Print and shaded views of the part. All mm, measured from the part's lowest x, y and z. A direction names the side the tool comes from. Give positions to 0.01 mm unless a question says otherwise; leave off trailing zeros. Order: outer loops, then holes, each group sorted by start corner. A loop starts at its lowest first (then second) coordinate and runs counter-clockwise, first axis right, second up. Notation, with made-up numbers: (10.5, -3.5) - (46.5, -3.5) arc R21 ccw to (46.5, 25.5) - close; hole circle Ø7 at (16, -36). An arc over 180 degrees is marked (long way). Answer in a Markdown table with one row per item.
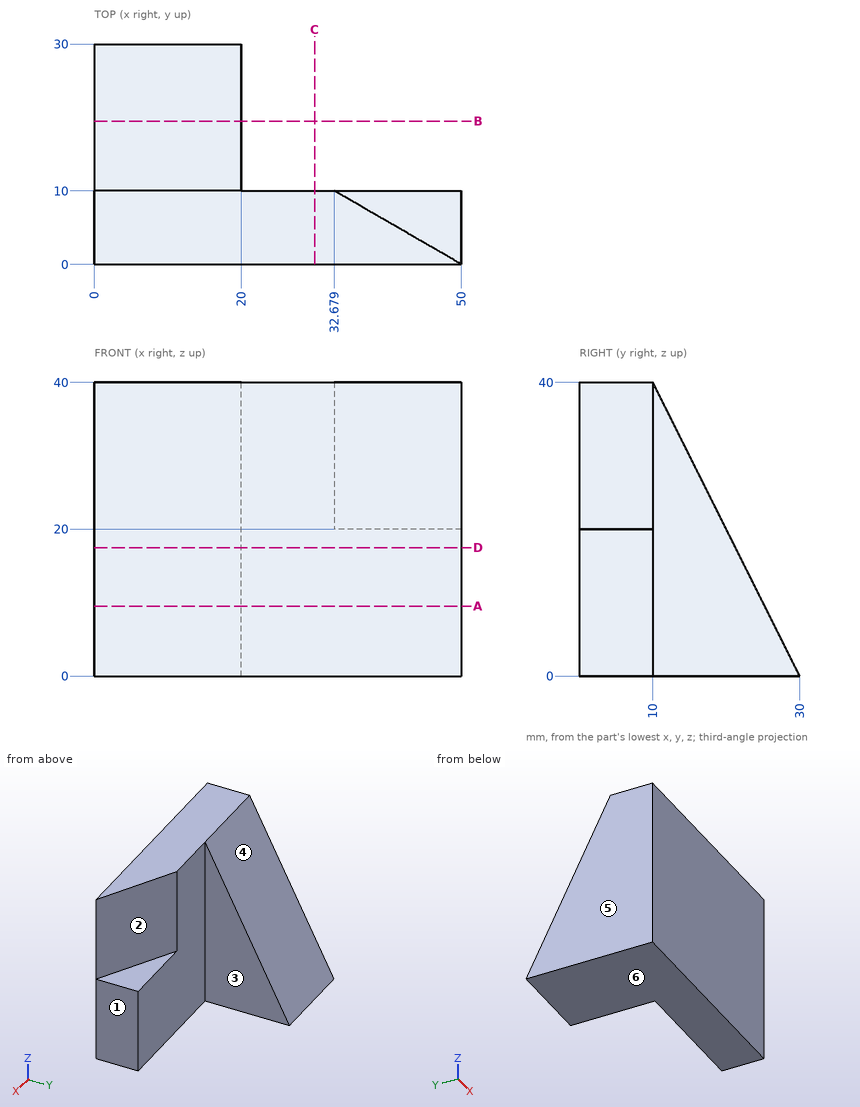
1. Cut at B-B on y = 19.5. Write the cut outline in (x, z), and give its area (3 significant figures).
Check result:
| item | result |
|---|---|
| outline | (0, 0) - (20, 0) - (20, 21) - (0, 21) - close |
| area | 420 mm² |
2. Drop flat-ended pins along their axis: P1, Ø6, axis at y = 16, z = 19.5, coming from the +X side; P2, Ø4, axis at x = 9.5, y = 15, coming from the +Z side; P3, Ø1, axis at x = 32, z = 18, coming from the +Y side. Give the stop position or say it passes through.
Check result:
| item | result |
|---|---|
| P1 | stops at x = 20 |
| P2 | stops at z = 34 |
| P3 | stops at y = 10 |
3. Cut at C-C on x = 30. Write the cut outline in (y, z), and give its area (3 significant figures).
Check result:
| item | result |
|---|---|
| outline | (0, 0) - (10, 0) - (10, 40) - (0, 40) - close |
| area | 400 mm² |
4. Which spindle directions (+Z, -Z, +X, -X, +Y, -Y) get a long thin tool onto all of the face, cutting with end or side? Do the marked faces 1, 2 and 3. Say none if no direction does.
Check result:
| item | result |
|---|---|
| face 1 | +Z, -Z, +X, +Y, -Y |
| face 2 | +Z, +X, +Y |
| face 3 | +Z, -Z, +X, +Y |
5. Probe line 1 (Y direction, x = 30, z = 10.5); line 2 (X direction, y = 23.5, z = 9.5); line 3 (Y direction, x = 39, z = 30). List the from-to ranges inside material, lowest first.
Check result:
| item | result |
|---|---|
| line 1 | y = 0 to 10 |
| line 2 | x = 0 to 20 |
| line 3 | y = 0 to 6.35 |
6. Cut at A-A on z = 9.5. Write the cut outline in (x, y).
Check result:
| item | result |
|---|---|
| outline | (0, 0) - (50, 0) - (50, 10) - (20, 10) - (20, 25.25) - (0, 25.25) - close |
7. Cut at D-D on z = 17.5. Write the cut outline in (x, y), and give its area (3 significant figures).
Check result:
| item | result |
|---|---|
| outline | (0, 0) - (50, 0) - (50, 10) - (20, 10) - (20, 21.25) - (0, 21.25) - close |
| area | 725 mm² |
8. Two-plate mould, pull along Z, no slides. Class the marked faces 4, 5 and 6: +Z half, -Z half, draft (parallel to the pull), parting line (faces both ways), or undercut.
Check result:
| item | result |
|---|---|
| face 4 | +Z half |
| face 5 | draft |
| face 6 | -Z half |
